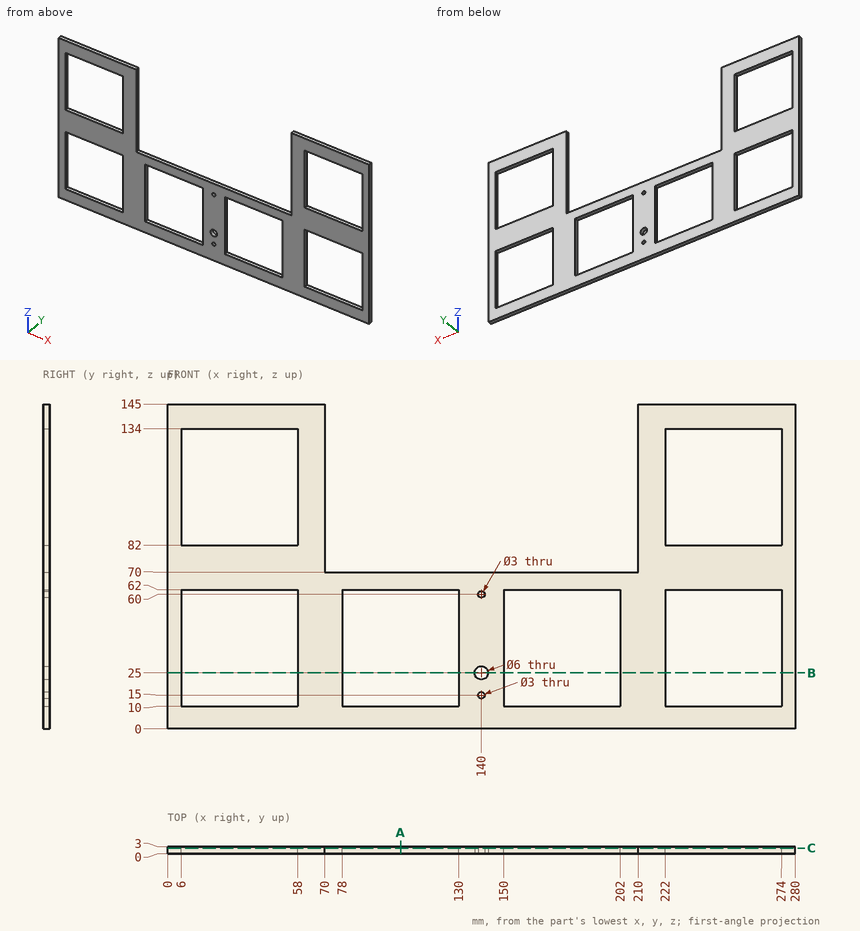
Input: dimensioned drawing with shaded views. Units: mm. Origin: part minimum x, y, z. Coordinates: 2 decimals unless noted, no trailing zeros. Order: outer loops, then holes, each group sorted by start corner. A loop starts at its lowest first (then second) coordinate and runs counter-clockwise, first axis right, second up.
1. Cut plane B-B, the plane z = 25. Return loops of the section in (x, y).
Checked values:
outline: (0, 0) - (6, 0) - (6, 3) - (0, 3) - close; (58, 0) - (78, 0) - (78, 3) - (58, 3) - close; (130, 0) - (137, 0) - (137, 3) - (130, 3) - close; (143, 0) - (150, 0) - (150, 3) - (143, 3) - close; (202, 0) - (222, 0) - (222, 3) - (202, 3) - close; (274, 0) - (280, 0) - (280, 3) - (274, 3) - close
2. Cut plane A-A, the plane x = 104. Return loops of the section in (y, z), plus the area to 3 significant figures.
Checked values:
outline: (0, 0) - (3, 0) - (3, 10) - (0, 10) - close; (0, 62) - (3, 62) - (3, 70) - (0, 70) - close
area: 54.0 mm2
3. Cut plane C-C, the plane y = 2.45. Count the separate pieces of the cut face and the enclosed holes in it, plus the area to 3 significant figures.
Checked values:
separate pieces: 1
enclosed holes: 9
area: 13,800 mm2
4. Contact query for a flat-ended pin moving along its axis: P1, Ø1.5, axis at x = 165.5, y = 1, coming from the +Z side. Output: stop coordinate, or through.
Checked values:
P1: stops at z = 70
5. Ray query, line 1 along X through (y, z) = (1.7, 105.5); line 2 along X through (y, z) = (0.9, 55.5); line 3 along X through (y, z) = (2.05, 60). Return the intervals inside material, ascending.
Checked values:
line 1: x = 0 to 6, 58 to 70, 210 to 222, 274 to 280
line 2: x = 0 to 6, 58 to 78, 130 to 150, 202 to 222, 274 to 280
line 3: x = 0 to 6, 58 to 78, 130 to 138.5, 141.5 to 150, 202 to 222, 274 to 280
